Model file for the job. Use its own axes, mm. Face numbers are marked on the shaded views. A direction names the side the tool comes from. Give positions to 0.01 mm unless a question says otherwise; leave off trailing zeros. Loops run counter-clockwise (first coordinate to the right, second up) from the corner with the lowest first, then second, coordinate; pieces in that order, holes last. Notation, with made-up numbers: (17.25, 73.5) -> (53.25, 73.5) arc R35 ccw to (53.25, 107.5) -> close; hole circle Ø3 at (59.5, -31.75). An arc over 180 degrees is marked (long way). Use CSV: the item, a comma, the result in double quotes. Start each with the question number.
(1) Cut at A-A on y = 33.5. Write the cut outline in (x, z).
(2) Drill centre lines: probe 1 along Z at (x, y) = (0.5, 27); probe 2 along Y at (x, z) = (7.5, -11); probe 3 along Y at (x, z) = (-10, 12.5). Where is each one in solid material? Low to high.
(3) Flat gauge pins, fed straight in: pin 1 (6 mm diameter, centred on y = 49.5, z = 13.5, fed in from +X); pin 2 (8 mm diameter, centred on y = 7, z = 13, fed in from -X); pin 3 (2 mm diameter, centred on y = 48, z = 8.5, fed in from +X). Where does each tip first touch, or does it go through?
(4) Cut at B-B on y = -4. Write the cut outline in (x, z), then the cut area to 3 significant figures.
(5) 3-axis set-ups, long thin cutter, end or side, ignore diameter. For the marked faces 1, 2 and 3: which of +Z, -Z, +X, -X, +Y, -Y reach the whole face in a straight line?
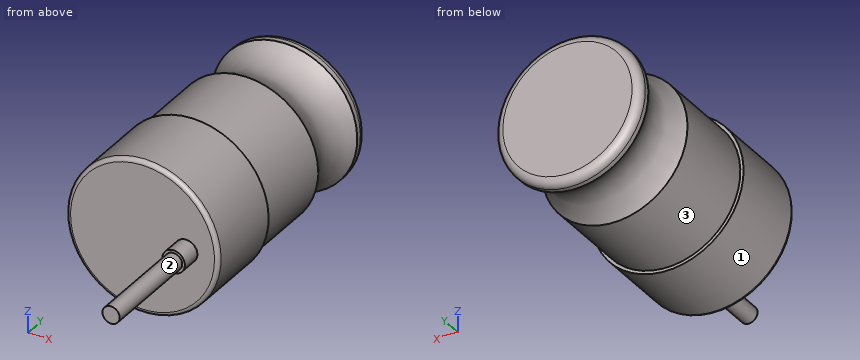
from build123d import *

# Parameters (mm, degrees)
SKETCH1_R           = 18.5
BOSS_EXTRUDE1_DEPTH = 20
SKETCH2_R           = 17.708290072
BOSS_EXTRUDE2_DEPTH = 40
SKETCH3_R           = 2.093314986
BOSS_EXTRUDE3_DEPTH = 30
FILLET1_R           = 2
FILLET2_R           = 1
SKETCH5_R           = 2.748707601
BOSS_EXTRUDE4_DEPTH = 5


with BuildPart() as part:
    # Sketch1 → Boss-Extrude1 (new body)
    with BuildSketch(Plane(origin=(0, 0, 0), x_dir=(1, 0, 0), z_dir=(0, 1, 0))):
        with Locations(Location((0, 0, 0), (0, 0, 270))):
            Circle(SKETCH1_R)
    extrude(amount=BOSS_EXTRUDE1_DEPTH)

    # Sketch2 → Boss-Extrude2 (add)
    with BuildSketch(Plane(origin=(0, 20, 0), x_dir=(1, 0, 0), z_dir=(0, 1, 0))):
        with Locations(Location((0, 0, 0), (0, 0, 270))):
            Circle(SKETCH2_R)
    extrude(amount=BOSS_EXTRUDE2_DEPTH)

    # Sketch3 → Boss-Extrude3 (add)
    with BuildSketch(Plane.XZ):
        with Locations(Location((10.583651539, 0, 0), (0, 0, 90))):
            Circle(SKETCH3_R)
    extrude(amount=BOSS_EXTRUDE3_DEPTH)

    # Sketch4 → Cut-Revolve1 (revolve, cut)
    with BuildSketch(Plane(origin=(0, 0, 0), x_dir=(0, 0, -1), z_dir=(1, 0, 0))):
        with BuildLine():
            add(Edge.make_bspline(
                [(-17.708290072, 56.753435872), (-12.088729605, 49.239761399), (-17.708290072, 41.11831897)],
                knots=[0, 0, 0, 1, 1, 1], degree=2))
            Line((-17.708290072, 41.11831897), (-17.708290072, 56.753435872))
        make_face()
    revolve(axis=Axis((0, 60, 0), (0, -1, 0)), mode=Mode.SUBTRACT)

    # Fillet1
    fillet1_edges = [part.edges().sort_by_distance(p)[0] for p in [
        (0, 60, -17.708290072),
    ]]
    fillet(fillet1_edges, radius=FILLET1_R)

    # Fillet2
    fillet2_edges = [part.edges().sort_by_distance(p)[0] for p in [
        (0, 0, -18.5),
    ]]
    fillet(fillet2_edges, radius=FILLET2_R)

    # Sketch5 → Boss-Extrude4 (add)
    with BuildSketch(Plane.XZ):
        with Locations(Location((10.583651539, 0, 0), (0, 0, 90))):
            Circle(SKETCH5_R)
    extrude(amount=BOSS_EXTRUDE4_DEPTH)


solid = part.part
Check result:
1,outline,"circle Ø35.42 at (0, 0)"
2,probe 1,"-17.7 to 17.7"
2,probe 2,"0 to 60"
2,probe 3,"0 to 44.12, 53.94 to 59.98"
3,pin 1,"x = 10.59"
3,pin 2,"x = -16.16"
3,pin 3,"x = 12.95"
4,outline,"circle Ø5.5 at (10.58, 0)"
4,area,"23.7 mm²"
5,face 1,"+Y, -Y"
5,face 2,"-Y"
5,face 3,"+Y"
